Autodesk Inventor part; units mm, degrees
ref_plane "YZ Plane" through (0, 0, 0) normal (1, 0, 0) x (0, 1, 0)
ref_plane "XY Plane" through (0, 0, 0) normal (0, 0, 1) x (1, 0, 0)
sketch "Sketch1" plane through (0, 0, 0) normal (0, 1, 0) x (-1, 0, 0)
  line L0 (12.7, 12.7) -> (-12.7, 12.7)
  line L1 (-12.7, 12.7) -> (-12.7, -12.7)
  line L2 (-12.7, -12.7) -> (12.7, -12.7)
  line L3 (12.7, -12.7) -> (12.7, 12.7)
  line L4 (12.7, 12.7) -> (-12.7, -12.7) construction
  line L5 (-12.7, 12.7) -> (12.7, -12.7) construction
  line L6 (9.525, 9.525) -> (-9.525, 9.525)
  line L7 (-9.525, 9.525) -> (-9.525, -9.525)
  line L8 (-9.525, -9.525) -> (9.525, -9.525)
  line L9 (9.525, -9.525) -> (9.525, 9.525)
  line L10 (9.525, 9.525) -> (-9.525, -9.525) construction
  line L11 (-9.525, 9.525) -> (9.525, -9.525) construction
  point P0 (0, 0)
  dimension "d0" = 25.4
  dimension "d1" = 3.175
extrude "Extrusion1" add sketch "Sketch1" along normal blind 1143
sketch "Sketch2" plane through (-12.7, 0, -12.7) normal (-1, 0, 0) x (0, 0, 1)
  point P0 (12.7, 0)
equation "\"d0\" = tubeSize"
equation "\"d1\" = tubeThickness"
equation "\"d2\" = tubeLength"
equation "\"tubeSize\" = 25.4"
equation "\"tubeThickness\" = 3.175"
equation "\"tubeLength\" = 1143"
properties part number "1_000_inchSquareTube" material "Aluminum 6061"
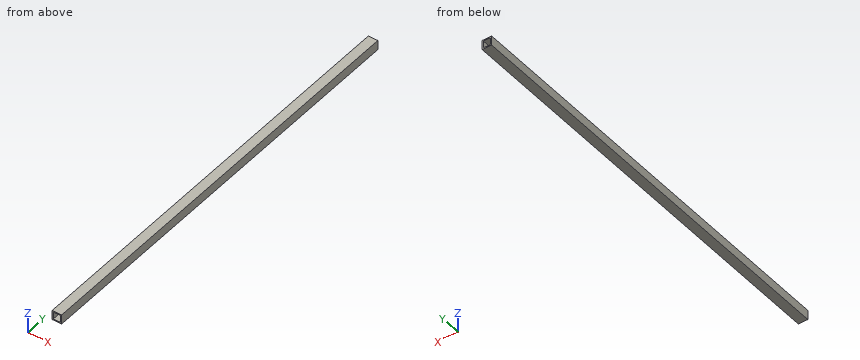
Read the model definition and answer for the solid it produces. Units are mm, in the model's axes. Round coordinates to 2 decimals unless told otherwise and drop trailing zeros. Write each loop counter-clockwise with the first axis right and the second up, starting at its lowest first coordinate (ties: lowest second). Pieces come first, ordered by that corner, then holes. Notation, with made-up numbers: M -22.75,61 L 28.25,61 A29 ccw 28.25,84 Z; hole C 50.25,71.5 d7. An arc over 180 degrees is marked long. Use a Markdown table: item, result.
1) The part is cut by section C-C (y = 872). Write down the section's boundary in (x, z) (3 decimals).
Answers follow:
| item | result |
|---|---|
| outline | M -12.7,-12.7 L 12.7,-12.7 L 12.7,12.7 L -12.7,12.7 Z; hole M -9.525,-9.525 L 9.525,-9.525 L 9.525,9.525 L -9.525,9.525 Z |
2) The part is cut by section B-B (x = -3.5). Write down the section's boundary in (y, z) (3 decimals), plus the area to 3 significant figures.
Answers follow:
| item | result |
|---|---|
| outline | M 0,-12.7 L 1143,-12.7 L 1143,-9.525 L 0,-9.525 Z; M 0,9.525 L 1143,9.525 L 1143,12.7 L 0,12.7 Z |
| area | 7,260 mm2 |
3) The part is cut by section A-A (z = 2.75). Write down the section's boundary in (x, y) (3 decimals).
Answers follow:
| item | result |
|---|---|
| outline | M -12.7,0 L -9.525,0 L -9.525,1143 L -12.7,1143 Z; M 9.525,0 L 12.7,0 L 12.7,1143 L 9.525,1143 Z |
4) A straight line is drawn through the part: line 1 along Z through (x, y) = (-6.75, 918.5) (3 decimals). Find the intervals that lie inside material, in ascending order. Write a range as [from, to].
Answers follow:
| item | result |
|---|---|
| line 1 | z = [-12.7, -9.525], [9.525, 12.7] |
5) A flat-ended cylindrical pin translates along its axis: pin 1 (1.5 mm diameter, centred on x = -5, z = 8.5, fed in from -Y). Find the tip coordinate at first contact, or state that the pin passes through.
Answers follow:
| item | result |
|---|---|
| pin 1 | passes through |
